Geometry: see drawing. Coordinates: mm, zero at the bounding-box minimum. A direction names the side the tool comes from. Give positions to 0.01 mm unless a question says otherwise; leave off trailing zeros. Loops run counter-clockwise (first coordinate to the right, second up) from the corner with the lowest first, then second, coordinate; pieces in that order, holes last. Notation, with made-up numbers: M 64,-21.5 L 104,-21.5 A9 cw 104,-4.5 Z; hole C -40,36 d9. An arc over 180 degrees is marked long. Answer in a Markdown table with one row per item.
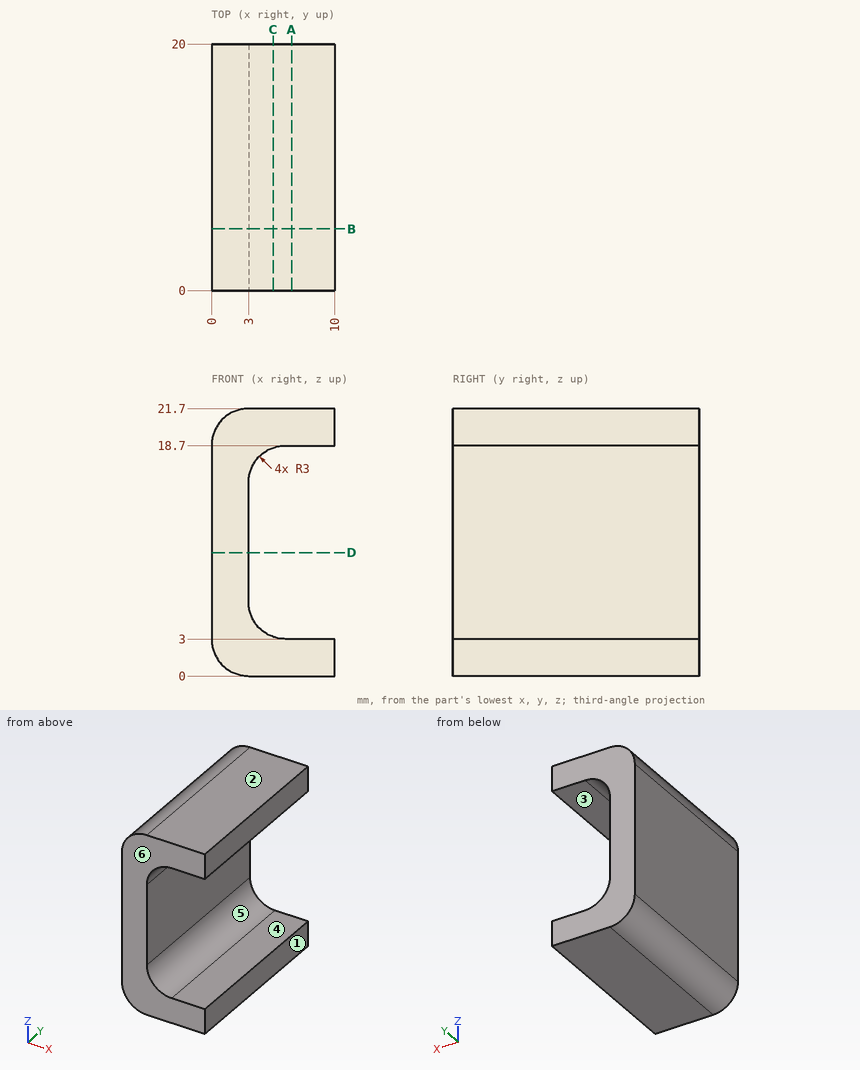
1) Section C-C, the plane x = 5. Return loops of the section in (y, z).
Reply:
| item | result |
|---|---|
| outline | M 0,0 L 20,0 L 20,3.17 L 0,3.17 Z; M 0,18.53 L 20,18.53 L 20,21.7 L 0,21.7 Z |
2) Section D-D, the plane z = 10. Return loops of the section in (x, y), then the cut area to 3 significant figures.
Reply:
| item | result |
|---|---|
| outline | M 0,0 L 3,0 L 3,20 L 0,20 Z |
| area | 60.0 mm² |
3) Pull-direction query (Z, two-part tool) for the marked faces 1, 2, 3 and 4; classes: released by +Z, released by -Z, zero draft, split by the parting line, or undercut.
Reply:
| item | result |
|---|---|
| face 1 | zero draft |
| face 2 | released by +Z |
| face 3 | undercut |
| face 4 | undercut |
4) Set-up query: the marked faces 5 and 6. Return all of +Z, -Z, +X, -X, +Y, -Y with unobstructed straight access to the full face (end or side cutting, diameter ignored); none if empty.
Reply:
| item | result |
|---|---|
| face 5 | +X, +Y, -Y |
| face 6 | +Z, -Z, +X, -X, -Y |
5) Pin query (flat end, axial travel): pin 1 Ø5 at (y, z) = (9, 9) entering from +X; pin 2 Ø1.5 at (x, z) = (4.5, 3.5) entering from +Y; pin 3 Ø2 at (x, z) = (8, 17) entering from -Y. Return the tip coordinate at first contact, or that it passes through.
Reply:
| item | result |
|---|---|
| pin 1 | stops at x = 3 |
| pin 2 | stops at y = 20 |
| pin 3 | passes through |
6) Section A-A, the plane x = 6.5. Return loops of the section in (y, z), then the cut area to 3 significant figures.
Reply:
| item | result |
|---|---|
| outline | M 0,0 L 20,0 L 20,3 L 0,3 Z; M 0,18.7 L 20,18.7 L 20,21.7 L 0,21.7 Z |
| area | 120 mm² |
7) Section B-B, the plane y = 5. Return loops of the section in (x, z), then the cut area to 3 significant figures.
Reply:
| item | result |
|---|---|
| outline | M 0,3 A3 ccw 3,0 L 10,0 L 10,3 L 6,3 A3 cw 3,6 L 3,15.7 A3 cw 6,18.7 L 10,18.7 L 10,21.7 L 3,21.7 A3 ccw 0,18.7 Z |
| area | 107 mm² |
8) Material intervals for L1, parallel to Z at x = 7, y = 7; L2, parallel to X at y = 12, z = 7.5; L3, parallel to Z at x = 4, y = 1.5, sorted ascending.
Reply:
| item | result |
|---|---|
| L1 | z = 0 to 3, 18.7 to 21.7 |
| L2 | x = 0 to 3 |
| L3 | z = 0 to 3.76, 17.94 to 21.7 |
